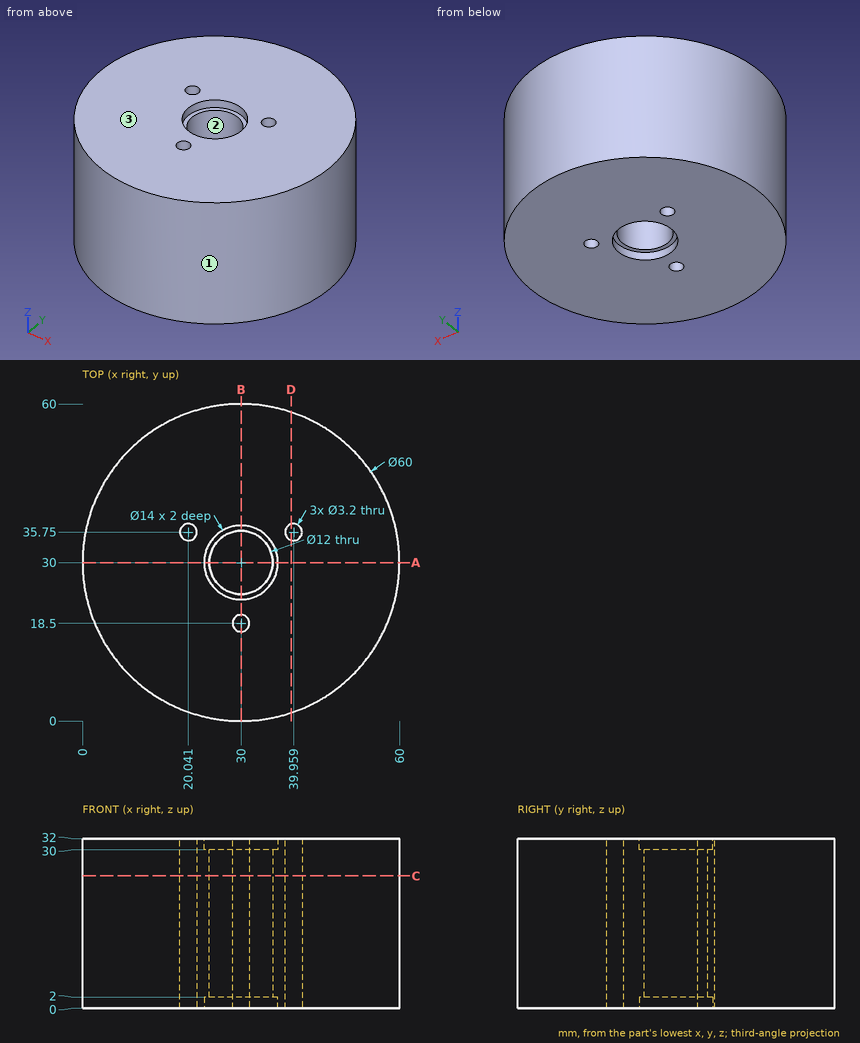
Can you work these out from the drawing? Everything is in mm from the part's minimum corner. Round coordinates to 2 decimals unless told otherwise and drop trailing zeros. Order: outer loops, then holes, each group sorted by start corner. A loop starts at its lowest first (then second) coordinate and runs counter-clockwise, first axis right, second up. Notation, with made-up numbers: M 88,9 L 100,9 A22 ccw 100,17 Z; hole C 55,-1.5 d2. An arc over 180 degrees is marked long. One line per question, with ' | ' between items.
1) I want a section at B-B, the plane x = 30. Write out the boundary of the cut face in (y, z), then the cut area to 3 significant figures.
Working result:
outline: M 0,0 L 16.9,0 L 16.9,32 L 0,32 Z; M 20.1,0 L 23,0 L 23,2 L 24,2 L 24,30 L 23,30 L 23,32 L 20.1,32 Z; M 36,2 L 37,2 L 37,0 L 60,0 L 60,32 L 37,32 L 37,30 L 36,30 Z | area: 1,430 mm²
2) I want a section at A-A, the plane y = 30. Write out the boundary of the cut face in (x, z), then the cut area to 3 significant figures.
Working result:
outline: M 0,0 L 23,0 L 23,2 L 24,2 L 24,30 L 23,30 L 23,32 L 0,32 Z; M 36,2 L 37,2 L 37,0 L 60,0 L 60,32 L 37,32 L 37,30 L 36,30 Z | area: 1,530 mm²
3) I need wall thicknesses on line 1 along Y through (x, z) = (30, 12.75); line 2 along X through (y, z) = (37, 15); line 3 along Y through (x, z) = (30, 31). Which ranges of each line are inside material? Lowest first, please.
Working result:
line 1: 0 to 16.9, 20.1 to 24, 36 to 60 | line 2: 0.83 to 19.04, 21.04 to 38.96, 40.96 to 59.17 | line 3: 0 to 16.9, 20.1 to 23, 37 to 60
4) For pin 1 Ø10 at (x, z) = (51, 25.5) entering from -Y; pin 2 Ø9.5 at (x, y) = (30, 30) entering from -Z; pin 3 Ø7 at (x, y) = (26.5, 31.5) entering from -Z; pin 4 Ø1 at (y, z) = (27.5, 16) entering from -X, each with a flat end and sliding along its axis, tell me the tip position at first contact or that it passes through.
Working result:
pin 1: y = 4.62 | pin 2: through | pin 3: z = 0 | pin 4: x = 0.07
5) I want a section at C-C, the plane z = 25. Write out the boundary of the cut face in (x, y).
Working result:
outline: C 30,30 d60; hole C 20.04,35.75 d3.2; hole C 30,30 d12; hole C 30,18.5 d3.2; hole C 39.96,35.75 d3.2
6) I want a section at D-D, the plane x = 39.5. Write out the boundary of the cut face in (y, z).
Working result:
outline: M 1.54,0 L 34.22,0 L 34.22,32 L 1.54,32 Z; M 37.28,0 L 58.46,0 L 58.46,32 L 37.28,32 Z
7) If we mould it in two halves opening along Y, with no side actions, what happens to the marked faces 1, 2 and 3? For each: +Y half, -Y half, draft (parallel to the pull), parting line (faces both ways), or undercut.
Working result:
face 1: parting line | face 2: undercut | face 3: draft
